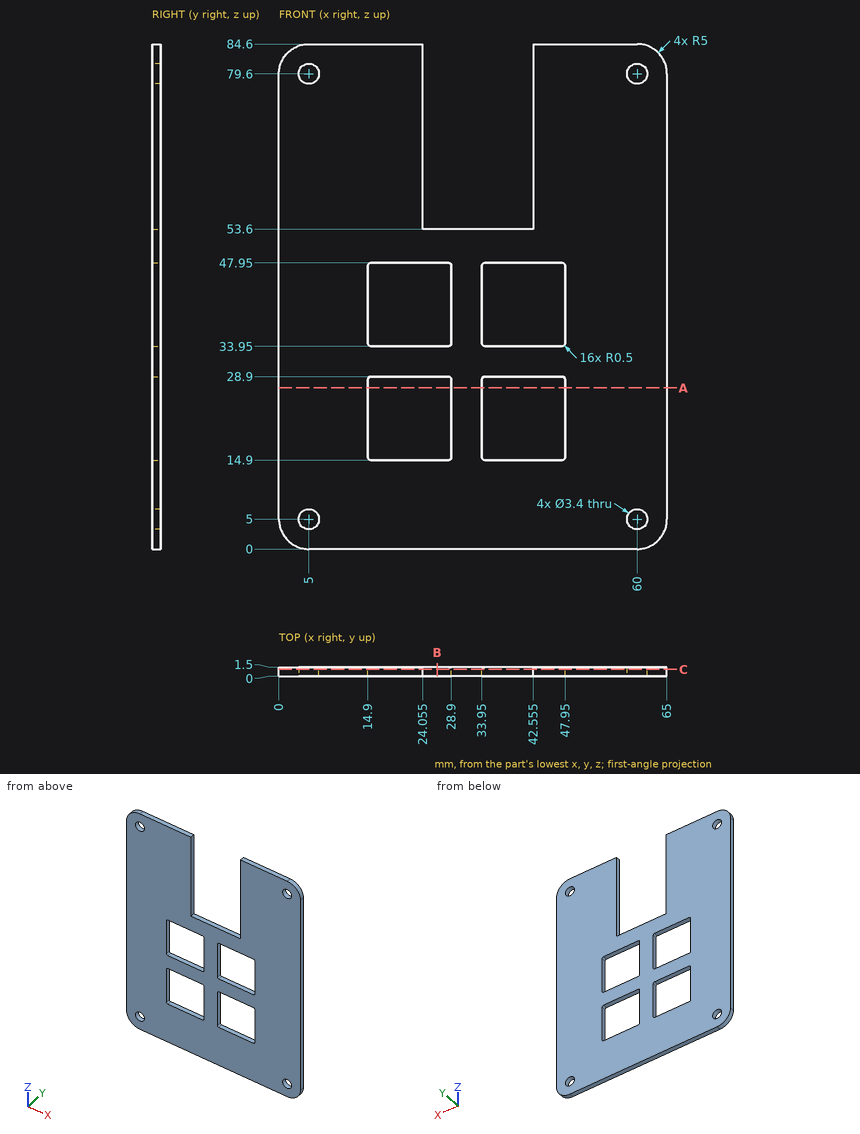
Here's the drawing with two shaded views (mm, measured from the low corner). I have some questions. Coordinates: 2 decimals unless noted, no trailing zeros. Write each loop counter-clockwise with the first axis right and the second up, starting at its lowest first coordinate (ties: lowest second). Pieces come first, ordered by that corner, then holes. Notation, with made-up numbers: (-16.5, 31.25) -> (17.5, 31.25) arc R15 cw to (17.5, 54.25) -> close; hole circle Ø11 at (72, 61). An arc over 180 degrees is marked (long way). Write item = value, one per line. Start each with the question number.
(1) I need wall thicknesses on line 1 (X direction, y = 1.2, z = 43.5); line 2 (Z direction, x = 42.5, y = 0.9); line 3 (Z direction, x = 60, y = 1.25). Which ranges of each line are inside material? Lowest first, please. Write a range as [from, to].
(2) I want a section at A-A (z = 27). Please give me the cut outline in (x, y).
(3) I want a section at C-C (y = 1.1). Give the number of separate pieces and of enclosed holes in the cut face, plus the area to 3 significant figures.
(4) I want a section at B-B (x = 26.5). Please give me the cut outline in (y, z).
Result set:
q1.line_1 = [0, 14.9], [28.9, 33.95], [47.95, 65]
q1.line_2 = [0, 14.9], [28.9, 33.95], [47.95, 53.6]
q1.line_3 = [0, 3.3], [6.7, 77.9], [81.3, 84.6]
q2.outline = (0, 0) -> (14.9, 0) -> (14.9, 1.5) -> (0, 1.5) -> close; (28.9, 0) -> (33.95, 0) -> (33.95, 1.5) -> (28.9, 1.5) -> close; (47.95, 0) -> (65, 0) -> (65, 1.5) -> (47.95, 1.5) -> close
q3.separate_pieces = 1
q3.enclosed_holes = 8
q3.area = 4,080 mm2
q4.outline = (0, 0) -> (1.5, 0) -> (1.5, 14.9) -> (0, 14.9) -> close; (0, 28.9) -> (1.5, 28.9) -> (1.5, 33.95) -> (0, 33.95) -> close; (0, 47.95) -> (1.5, 47.95) -> (1.5, 53.6) -> (0, 53.6) -> close
